from build123d import *

# Parameters (mm, degrees)
SALIENTE_EXTRUIR1_DEPTH = 62
CORTAR_EXTRUIR1_DEPTH   = 20
CORTAR_EXTRUIR2_START   = 25
CORTAR_EXTRUIR2_DEPTH   = 124
CORTAR_EXTRUIR3_DEPTH   = 3.901378
REDONDEO1_R             = 10


with BuildPart() as part:
    # Croquis1 → Saliente-Extruir1 (new body, symmetric)
    with BuildSketch(Plane.XY):
        with BuildLine():
            Line((0, 0), (0, 75))
            ThreePointArc((0, 75), (3.711686747, 79.831174698), (9.336099585, 77.489626556))
            ThreePointArc((9.336099585, 77.489626556), (24.745312475, 40.098749993), (30, 0))
            Line((30, 0), (0, 0))
        make_face()
    extrude(amount=SALIENTE_EXTRUIR1_DEPTH, both=True)

    # Croquis3 → Cortar-Extruir1 (cut, symmetric)
    with BuildSketch(Plane.XY):
        Polygon((9.336099585, 77.489626556), (4, 62.828813438), (4, 4), (29.948585885, 4), (32.228439928, 77.489626556), align=None)
    extrude(amount=CORTAR_EXTRUIR1_DEPTH, both=True, mode=Mode.SUBTRACT)

    # Croquis4 → Cortar-Extruir2 (cut)
    with BuildSketch(Plane.XY.offset(CORTAR_EXTRUIR2_START)):
        Polygon((9.336099585, 77.489626556), (4, 62.828813438), (4, 3.901378225), (34.928853612, 3.901378225), (21.567933324, 77.489626556), align=None)
    cortar_extruir2 = extrude(amount=CORTAR_EXTRUIR2_DEPTH, mode=Mode.SUBTRACT)

    # Simetría1: Cortar-Extruir2 across plane
    add(cortar_extruir2.mirror(Plane.XY), mode=Mode.SUBTRACT)

    # Croquis5 → Cortar-Extruir3 (cut)
    with BuildSketch(Plane.XZ):
        with BuildLine():
            Line((10, 30.6), (20, 30.6))
            ThreePointArc((20, 30.6), (21.6, 29), (20, 27.4))
            Line((20, 27.4), (10, 27.4))
            ThreePointArc((10, 27.4), (8.4, 29), (10, 30.6))
        make_face()
        with BuildLine():
            Line((10, -30.6), (20, -30.6))
            ThreePointArc((20, -30.6), (21.6, -29), (20, -27.4))
            Line((20, -27.4), (10, -27.4))
            ThreePointArc((10, -27.4), (8.4, -29), (10, -30.6))
        make_face()
    extrude(amount=-CORTAR_EXTRUIR3_DEPTH, mode=Mode.SUBTRACT)

    # Redondeo1
    redondeo1_edges = [part.edges().sort_by_distance(p)[0] for p in [
        (29.987772095, 1.950842396, -62),
        (29.987772095, 1.950842396, 62),
    ]]
    fillet(redondeo1_edges, radius=REDONDEO1_R)


solid = part.part
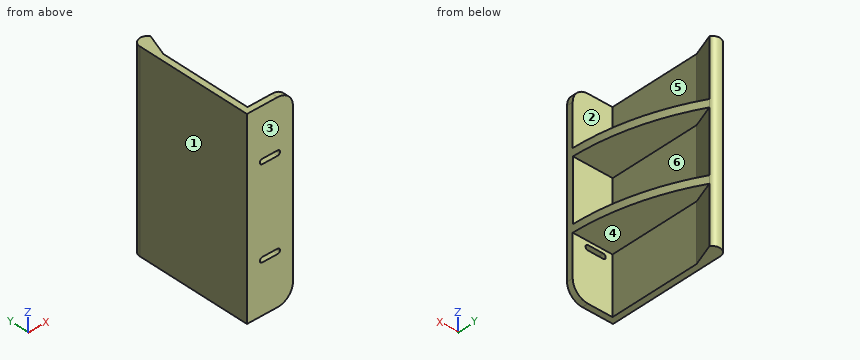
Source: CAD feature listing. Evaluate the final solid. Frame: model axes, mm. Face numbers are marked on the shaded views. A direction names the side the tool comes from. Give positions to 0.01 mm unless a question says otherwise; leave off trailing zeros. Write each loop counter-clockwise with the first axis right and the second up, starting at its lowest first coordinate (ties: lowest second). Pieces come first, ordered by that corner, then holes. Notation, with made-up numbers: M 30,-9 L 75,-9 A26 ccw 75,11 Z; hole C 34,65.25 d7. An arc over 180 degrees is marked long. Return JSON: item names as keys, results as strings. Group by question number.
1) Draft query along Y for the marked faces 1, 2 and 3. Return one class per face: released by +Y, released by -Y, zero draft, split by the parting line, or undercut.
2) Ray query, L1, parallel to Z at x = 11.5, y = 48; L2, parallel to Y at x = 13.5, z = 16. Return the intervals inside material, ascending.
3) Cut plane D-D, the plane y = 21.5. Output: boundary loops of the cut face in (x, z), then the cut area to 3 significant figures.
4) First-contact query: pin 1 Ø5 at (x, y) = (15, 62) entering from -Z; pin 2 Ø4 at (x, z) = (19, -6) entering from -Y; pin 3 Ø12 at (x, y) = (23, 44.5) entering from +Z; pin 4 Ø11 at (y, z) = (21, 45.5) entering from +X. Flat tips, straight axial feed; report the tip coordinate or a pass-through.
5) Set-up query: the marked faces 4, 5 and 6. Return all of +Z, -Z, +X, -X, +Y, -Y with unobstructed straight access to the full face (end or side cutting, diameter ignored); none if empty.
6) Cut plane B-B, the plane z = -35. Output: boundary loops of the cut face in (x, y) (3 decimals), then the cut area to 3 significant figures.
7) Cut plane A-A, the plane z = 29. Output: boundary loops of the cut face in (x, y) (3 decimals), then the cut area to 3 significant figures.
8) Cut plane C-C, the plane y = 51.5. Output: boundary loops of the cut face in (x, z), then the cut area to 3 significant figures.
Data:
{
 "1": {"face 1": "zero draft", "face 2": "undercut", "face 3": "released by -Y"},
 "2": {"L1": "z = -25 to -20, 20 to 25", "L2": "y = 0 to 4"},
 "3": {"outline": "M 0,-62 L 4,-62 L 4,-25 L 28.51,-25 L 28.51,-20 L 4,-20 L 4,20 L 28.51,20 L 28.51,25 L 4,25 L 4,62 L 0,62 Z", "area": "741 mm²"},
 "4": {"pin 1": "stops at z = -25", "pin 2": "stops at y = 0", "pin 3": "stops at z = 25", "pin 4": "stops at x = 4"},
 "5": {"face 4": "-Z, +X", "face 5": "+Z, +X", "face 6": "+X"},
 "6": {"outline": "M 0,0 L 30,0 A155.625 ccw 29.951,3.901 L 4,3.901 L 4,62.829 L 9.336,77.49 A5 ccw 0,75 Z", "area": "465 mm²"},
 "7": {"outline": "M 0,0 L 8.4,0 L 8.4,3.901 L 4,3.901 L 4,62.829 L 9.336,77.49 A5 ccw 0,75 Z; M 21.6,0 L 30,0 A155.625 ccw 29.951,3.901 L 21.6,3.901 Z", "area": "414 mm²"},
 "8": {"outline": "M 0,-62 L 4,-62 L 4,-25 L 21.23,-25 L 21.23,-20 L 4,-20 L 4,20 L 21.23,20 L 21.23,25 L 4,25 L 4,62 L 0,62 Z", "area": "668 mm²"}
}
